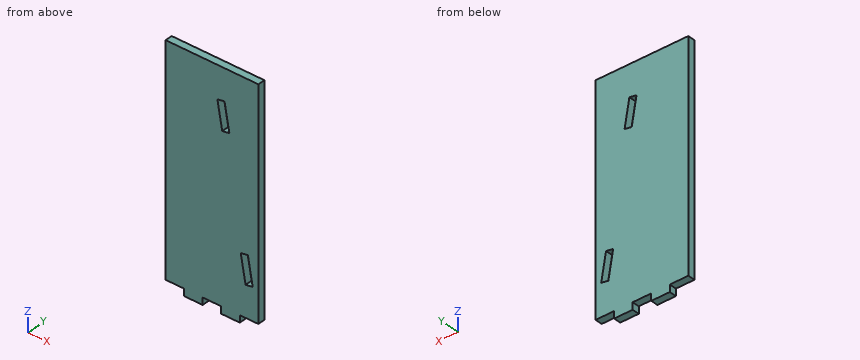
```python
from build123d import *

# Parameters (mm, degrees)
F0_W     = 50.8
F0_H     = 19.05
F1_DEPTH = 19.812


# Not quite as in the source:
# - a feature names something its author has since deleted; it is built from what else it names


with BuildPart() as f1:
    # F0 (on Front) → F1 (new body)
    with BuildSketch(Plane.XZ):
        Polygon((239.4815002712, 559.237990855), (-14.5184997288, 559.237990855), (-14.5184997288, -50.362009145), (36.2815002712, -50.362009145), (87.0815002712, -50.362009145), (137.8815002712, -50.362009145), (188.6815002712, -50.362009145), (219.3638682365, -50.362009145), (204.533166074, 33.7470824019), (191.3011749357, 108.7894331814), (140.5785422392, 396.4517778362), (127.346551101, 471.4941286158), (113.5079391308, 549.9767970912), (133.6255711655, 549.9767970912), (146.8575623037, 474.9344463117), (160.0895534419, 399.8920955322), (210.8121861384, 112.2297508773), (224.0441772766, 37.1874000978), (239.4815002712, -50.362009145), align=None)
        with Locations((61.6815002712, -59.887009145)):
            Rectangle(F0_W, F0_H)
        with Locations((163.2815002712, -59.887009145)):
            Rectangle(F0_W, F0_H)
        Polygon((127.346551101, 471.4941286158), (146.8575623037, 474.9344463117), (133.6255711655, 549.9767970912), (113.5079391308, 549.9767970912), align=None)
        Polygon((219.3638682365, -50.362009145), (239.4815002712, -50.362009145), (224.0441772766, 37.1874000978), (204.533166074, 33.7470824019), align=None)
        Polygon((191.3011749357, 108.7894331814), (210.8121861384, 112.2297508773), (160.0895534419, 399.8920955322), (140.5785422392, 396.4517778362), align=None)
    extrude(amount=F1_DEPTH)


solid = f1.part
```
The listing builds one solid part. Answer for the finished solid, in the listing's coordinates (mm). Round coordinates to 2 decimals unless told otherwise and drop trailing zeros. Order: outer loops, then holes, each group sorted by start corner. A loop starts at its lowest first (then second) coordinate and runs counter-clockwise, first axis right, second up. Notation, with made-up numbers: (5, 54.5) - (38, 54.5) arc R21 ccw to (38, 68.5) - close; hole circle Ø7 at (38, 43.5). An arc over 180 degrees is marked (long way). Put each result on its own line as item: value. Start each with the question number.
(1) Find section A-A (y = -16.75). Give the vertices of the cut face in (x, z), plus the area to 3 significant figures.
(2) Straight lines are drawn through the part: probe 1 along X at (y, z) = (-1.5, 43.5); probe 2 along X at (y, z) = (-7.5, 440.5); probe 3 along Z at (x, y) = (117, -4.5). For each, find the intervals that lie inside material, in ascending order. Write a range as from..to.
(3) Given P1, Ø3, axis at x = 90, y = -11, coming from the -Z side; P2, Ø5.5, axis at y = -8, z = -62, coming from the -X side, each flat-ended and moving along its own axis, determine where each tip first touches the part or whether it passes through.
(4) Find section B-B (z = 96). Give the vertices of the cut face in (x, y), plus the area to 3 significant figures.
(5) Find section C-C (x = 99.5). Give the vertices of the cut face in (y, z), plus the area to 3 significant figures.
Reply:
1. outline: (-14.52, -50.36) - (36.28, -50.36) - (36.28, -69.41) - (87.08, -69.41) - (87.08, -50.36) - (137.88, -50.36) - (137.88, -69.41) - (188.68, -69.41) - (188.68, -50.36) - (239.48, -50.36) - (239.48, 559.24) - (-14.52, 559.24) - close; hole (127.35, 471.49) - (140.58, 396.45) - (160.09, 399.89) - (146.86, 474.93) - close; hole (191.3, 108.79) - (204.53, 33.75) - (224.04, 37.19) - (210.81, 112.23) - close
1. area: 154,000 mm^2
2. probe 1: -14.52..202.81, 222.93..239.48
2. probe 2: -14.52..132.81, 152.93..239.48
2. probe 3: -50.36..559.24
3. P1: z = -50.36
3. P2: x = 36.28
4. outline: (-14.52, -19.81) - (193.56, -19.81) - (193.56, 0) - (-14.52, 0) - close; (213.67, -19.81) - (239.48, -19.81) - (239.48, 0) - (213.67, 0) - close
4. area: 4,630 mm^2
5. outline: (-19.81, -50.36) - (0, -50.36) - (0, 559.24) - (-19.81, 559.24) - close
5. area: 12,100 mm^2
